Here's how the part is built. I have some questions about the finished solid (model axes, mm). Round coordinates to 2 decimals unless told otherwise and drop trailing zeros. Order: outer loops, then holes, each group sorted by start corner. A loop starts at its lowest first (then second) coordinate and runs counter-clockwise, first axis right, second up. Notation, with made-up numbers: (65, 55.5) -> (86, 55.5) arc R25 cw to (86, 85.5) -> close; hole circle Ø11 at (69.25, 44.5). An arc over 180 degrees is marked (long way). Use a Markdown table: item, result. Add a question column.
(1) I want a section at B-B, the plane x = 21. Please give me the cut outline in (y, z), then the cut area to 3 significant figures.
(2) If I drill on probe 1 along X at (y, z) = (4.05, 10.5); probe 2 along Z at (x, y) = (0, 1.1); probe 3 along X at (y, z) = (2.45, -13), over which ranges is the centre line in solid material (lowest first)?
(3) I want a section at C-C, the plane y = 2.05. Give the number of separate pieces and of enclosed holes in the cut face, then the cut area to 3 significant figures.
(4) I want a section at A-A, the plane x = 0. Please give me the cut outline in (y, z), then the cut area to 3 significant figures.
(5) Thinking about a two-plate mould opening in Z: for faces 1 (the face through (-42.719, 2.282, 62.594)), 2 (the face through (-1, 4.5, 30)), 3 (the face through (38.1, 2.28, 5.86)), which applies, pulls with the +Z half, pulls with the -Z half, needs draft (parallel to the pull), parting line crosses it, or undercut?
from build123d import *

# Parameters (mm, degrees)
F0_W      = 90
F0_H      = 130
F1_DEPTH  = 4.5
F2_R      = 8
F3_R      = 28.625
F4_DEPTH  = 4.501
F5_R      = 1.625
F6_DEPTH  = 4.501
F7_R      = 1.25
F8_DEPTH  = 4.501
F9_W      = 7.5
F9_H      = 25
F10_DEPTH = 4.501
F11_R     = 3


with BuildPart() as f1:
    # F0 (on Front) → F1 (new body)
    with BuildSketch(Plane.XZ):
        Rectangle(F0_W, F0_H)
    extrude(amount=-F1_DEPTH)

    # F2
    f2_edges = [f1.edges().sort_by_distance(p)[0] for p in [
        (45, 2.25, 65),
        (45, 2.25, -65),
        (-45, 2.25, -65),
        (-45, 2.25, 65),
    ]]
    fillet(f2_edges, radius=F2_R)

    # F3 (on Front) → F4 (cut, through all)
    with BuildSketch(Plane.XZ):
        with Locations((0, -2.157351)):
            Circle(F3_R)
    extrude(amount=-F4_DEPTH, mode=Mode.SUBTRACT)

    # F5 (on Front) → F6 (cut, through all)
    with BuildSketch(Plane.XZ):
        with Locations((-37, 57)):
            Circle(F5_R)
        with Locations((37, 57)):
            Circle(F5_R)
        with Locations((-37, -57)):
            Circle(F5_R)
        with Locations((37, -57)):
            Circle(F5_R)
    extrude(amount=-F6_DEPTH, mode=Mode.SUBTRACT)

    # F7 (on Front) → F8 (cut, through all)
    with BuildSketch(Plane.XZ):
        with Locations((-25, 25)):
            Circle(F7_R)
        with Locations((25, 25)):
            Circle(F7_R)
        with Locations((-25, -25)):
            Circle(F7_R)
        with Locations((25, -25)):
            Circle(F7_R)
    extrude(amount=-F8_DEPTH, mode=Mode.SUBTRACT)

    # F9 (on Front) → F10 (cut, through all)
    with BuildSketch(Plane.XZ):
        Polygon((30, 50), (-30, 50), (-25, 35), (25, 35), align=None)
        with Locations((35.25, 17.5)):
            Rectangle(F9_W, F9_H)
        with Locations((35.25, -17.5)):
            Rectangle(F9_W, F9_H)
        Polygon((30, -50), (25, -35), (-25, -35), (-30, -50), align=None)
        with Locations((-35.25, -17.5)):
            Rectangle(F9_W, F9_H)
        with Locations((-35.25, 17.5)):
            Rectangle(F9_W, F9_H)
    extrude(amount=-F10_DEPTH, mode=Mode.SUBTRACT)

    # F11
    f11_edges = [f1.edges().sort_by_distance(p)[0] for p in [
        (-39, 2.25, 5),
        (-39, 2.25, -30),
        (-30, 2.25, -50),
        (-25, 2.25, 35),
        (31.5, 2.25, 5),
        (31.5, 2.25, -30),
        (39, 2.25, -30),
        (39, 2.25, 5),
        (25, 2.25, 35),
        (30, 2.25, -50),
        (39, 2.25, 30),
        (39, 2.25, -5),
        (25, 2.25, -35),
        (31.5, 2.25, -5),
        (31.5, 2.25, 30),
        (-30, 2.25, 50),
        (30, 2.25, 50),
        (-25, 2.25, -35),
        (-39, 2.25, -5),
        (-39, 2.25, 30),
        (-31.5, 2.25, 30),
        (-31.5, 2.25, -5),
        (-31.5, 2.25, -30),
        (-31.5, 2.25, 5),
    ]]
    fillet(f11_edges, radius=F11_R)


solid = f1.part
Taken from the geometry:
| question | item | result |
|---|---|---|
| 1 | outline | (0, -65) -> (4.5, -65) -> (4.5, -50) -> (0, -50) -> close; (0, -35) -> (4.5, -35) -> (4.5, -21.61) -> (0, -21.61) -> close; (0, 17.29) -> (4.5, 17.29) -> (4.5, 35) -> (0, 35) -> close; (0, 50) -> (4.5, 50) -> (4.5, 65) -> (0, 65) -> close |
| 1 | area | 275 mm2 |
| 2 | probe 1 | x = -45 to -39, -31.5 to -25.67, 25.67 to 31.5, 39 to 45 |
| 2 | probe 2 | z = -65 to -50, -35 to -30.78, 26.47 to 35, 50 to 65 |
| 2 | probe 3 | x = -45 to -39, -31.5 to -26.49, 26.49 to 31.5, 39 to 45 |
| 3 | separate pieces | 1 |
| 3 | enclosed holes | 15 |
| 3 | area | 6,670 mm2 |
| 4 | outline | (0, -65) -> (4.5, -65) -> (4.5, -50) -> (0, -50) -> close; (0, -35) -> (4.5, -35) -> (4.5, -30.78) -> (0, -30.78) -> close; (0, 26.47) -> (4.5, 26.47) -> (4.5, 35) -> (0, 35) -> close; (0, 50) -> (4.5, 50) -> (4.5, 65) -> (0, 65) -> close |
| 4 | area | 192 mm2 |
| 5 | face 1 | pulls with the +Z half |
| 5 | face 2 | needs draft |
| 5 | face 3 | undercut |
